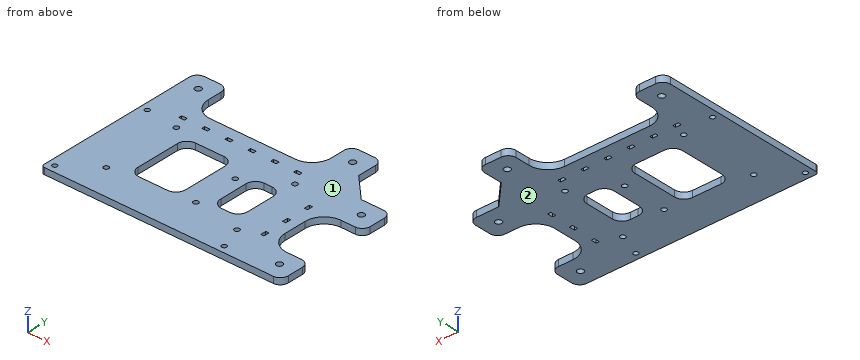
Autodesk Inventor part; units mm, degrees
ref_plane "YZ Plane" through (0, 0, 0) normal (1, 0, 0) x (0, 1, 0)
ref_plane "XZ Plane" through (0, 0, 0) normal (0, 1, 0) x (-1, 0, 0)
ref_plane "XY Plane" through (0, 0, 0) normal (0, 0, 1) x (1, 0, 0)
sketch "Szkic1" plane through (0, 0, 0) normal (0, 0, 1) x (1, 0, 0)
  line L0 (0, 53.1646) -> (0, 0)
  line L1 (0, 0) -> (98.9175, 0)
  line L2 (98.9175, 0) -> (98.9175, 1.2597)
  line L3 (98.9175, 1.2597) -> (101.455, 3.8466)
  line L4 (101.455, 3.8466) -> (101.455, 38.0126)
  line L5 (101.455, 38.0126) -> (98.9175, 40.5017)
  line L6 (98.9175, 40.5017) -> (98.9175, 50.7051)
  line L7 (98.9175, 50.7051) -> (96.4101, 53.1646)
  line L8 (96.4101, 53.1646) -> (0, 53.1646)
  circle A0 centre (96.3111, 2.4061) radius 1.6
  circle A1 centre (15.0311, 50.6661) radius 1.6
  circle A2 centre (89.9611, 50.6661) radius 1.6
  circle A3 centre (13.7611, 2.4061) radius 1.6
  circle A4 centre (65.8311, 35.4261) radius 1.6
  circle A5 centre (65.8311, 7.4861) radius 1.6
  line L9 (-10, 93.1646) -> (141.455, 93.1646)
  line L10 (141.455, 93.1646) -> (141.455, -17)
  line L11 (141.455, -17) -> (-10, -17)
  line L12 (-10, -17) -> (-10, 93.1646)
  line L13 (107.455, 93.1646) -> (107.455, 61.1646)
  line L14 (107.455, 61.1646) -> (141.455, 61.1646)
  point P0 (-10, 13.9306)
  point P1 (7.9866, -17)
  dimension "d0" = 101.455
  dimension "d1" = 53.1646
  dimension "d2" = 98.9175
  dimension "d3" = 15.0311
  dimension "d4" = 2.4986
  dimension "d5" = 3.2
  dimension "d6" = 2.4986
  dimension "d7" = 8.9564
  dimension "d8" = 3.2
  dimension "d9" = 3.2
  dimension "d10" = 17.7386
  dimension "d11" = 65.8311
  dimension "d12" = 13.7611
  dimension "d13" = 2.4061
  dimension "d14" = 7.486
  dimension "d15" = 65.8311
  dimension "d16" = 2.4061
  dimension "d17" = 5.144
  dimension "d18" = 3.2
  dimension "d19" = 3.2
  dimension "d20" = 3.2
  dimension "d21" = 98.9175
  dimension "d22" = 1.2597
  dimension "d23" = 10.2034
  dimension "d24" = 34.166
  dimension "d33" = 40
  dimension "d34" = 40
  dimension "d35" = 17
  dimension "d36" = 10
  dimension "d37" = 34
  dimension "d38" = 32
extrude "Wyciągnięcie proste1" add sketch "Szkic1" along normal blind 4 contours L8 L7 L6 L5 L4 L3 L2 L1 L0 | L9 L13 L14 L10 L11 L12
chamfer "Faza1" distance 15 angle 45 1 edges at (107.455, 61.1646, 2)
sketch "Szkic2" plane through (0, 0, 4) normal (0, 0, 1) x (1, 0, 0)
  circle A0 centre (65.8311, 7.4861) radius 1.6
  circle A1 centre (15.0311, 50.6661) radius 1.6
  circle A2 centre (89.9611, 50.6661) radius 1.6
  circle A3 centre (13.7611, 2.4061) radius 1.6
  circle A4 centre (65.8311, 35.4261) radius 1.6
  circle A5 centre (96.3111, 2.4061) radius 1.6
  line L0 (-10, 93.1646) -> (-10, -17)
  line L1 (-10, -17) -> (141.455, -17)
  line L2 (141.455, -17) -> (141.455, 61.1646)
  line L3 (141.455, 61.1646) -> (122.455, 61.1646)
  line L4 (107.455, 76.1646) -> (122.455, 61.1646)
  line L5 (107.455, 76.1646) -> (107.455, 93.1646)
  line L6 (107.455, 93.1646) -> (-10, 93.1646)
  line L7 (10, 93.1646) -> (10, 67.1646)
  line L8 (10, 67.1646) -> (87.455, 67.1646)
  line L9 (87.455, 67.1646) -> (87.455, 93.1646)
  line L10 (107.455, 93.1646) -> (-10, 93.1646)
  line L11 (141.455, -17) -> (141.455, 61.1646)
  line L12 (141.455, 41.1646) -> (115.455, 41.1646)
  line L13 (115.455, 41.1646) -> (115.455, 3)
  line L14 (115.455, 3) -> (141.455, 3)
  line L15 (10, 60.1646) -> (13.5, 60.1646)
  line L16 (13.5, 60.1646) -> (13.5, 58.1646)
  line L17 (13.5, 58.1646) -> (10, 58.1646)
  line L18 (10, 58.1646) -> (10, 60.1646)
  line L19 (28, 58.1646) -> (24.5, 58.1646)
  line L20 (28, 60.1646) -> (28, 58.1646)
  line L21 (24.5, 60.1646) -> (28, 60.1646)
  line L22 (24.5, 58.1646) -> (24.5, 60.1646)
  line L23 (42.5, 58.1646) -> (39, 58.1646)
  line L24 (42.5, 60.1646) -> (42.5, 58.1646)
  line L25 (39, 60.1646) -> (42.5, 60.1646)
  line L26 (39, 58.1646) -> (39, 60.1646)
  line L27 (57, 58.1646) -> (53.5, 58.1646)
  line L28 (57, 60.1646) -> (57, 58.1646)
  line L29 (53.5, 60.1646) -> (57, 60.1646)
  line L30 (53.5, 58.1646) -> (53.5, 60.1646)
  line L31 (71.5, 58.1646) -> (68, 58.1646)
  line L32 (71.5, 60.1646) -> (71.5, 58.1646)
  line L33 (68, 60.1646) -> (71.5, 60.1646)
  line L34 (68, 58.1646) -> (68, 60.1646)
  line L35 (86, 58.1646) -> (82.5, 58.1646)
  line L36 (86, 60.1646) -> (86, 58.1646)
  line L37 (82.5, 60.1646) -> (86, 60.1646)
  line L38 (82.5, 58.1646) -> (82.5, 60.1646)
  line L39 (109.455, 41.1646) -> (107.455, 41.1646)
  line L40 (107.455, 41.1646) -> (107.455, 37.6646)
  line L41 (107.455, 37.6646) -> (109.455, 37.6646)
  line L42 (109.455, 37.6646) -> (109.455, 41.1646)
  line L43 (107.455, 25.6646) -> (107.455, 22.1646)
  line L44 (107.455, 22.1646) -> (109.455, 22.1646)
  line L45 (109.455, 22.1646) -> (109.455, 25.6646)
  line L46 (109.455, 25.6646) -> (107.455, 25.6646)
  line L47 (107.455, 10.1646) -> (107.455, 6.6646)
  line L48 (107.455, 6.6646) -> (109.455, 6.6646)
  line L49 (109.455, 6.6646) -> (109.455, 10.1646)
  line L50 (109.455, 10.1646) -> (107.455, 10.1646)
  line L51 (54.7961, 6.5361) -> (24.7961, 6.5361)
  line L52 (24.7961, 6.5361) -> (24.7961, 46.5361)
  line L53 (24.7961, 46.5361) -> (54.7961, 46.5361)
  line L54 (54.7961, 46.5361) -> (54.7961, 6.5361)
  line L55 (89.5711, 11.5361) -> (72.5711, 11.5361)
  line L56 (72.5711, 11.5361) -> (72.5711, 41.5361)
  line L57 (72.5711, 41.5361) -> (89.5711, 41.5361)
  line L58 (89.5711, 41.5361) -> (89.5711, 11.5361)
  point P0 (0, 0)
  point P1 (131.455, -7)
  point P2 (131.455, 51.1646)
  point P3 (97.455, 83.1646)
  point P4 (0, 83.1646)
  dimension "d42" = 20
  dimension "d43" = 20
  dimension "d44" = 20
  dimension "d45" = 20
  dimension "d46" = 26
  dimension "d47" = 26
  dimension "d50" = 3.5
  dimension "d51" = 2
  dimension "d52" = 7
  dimension "d55" = 14.5
  dimension "d62" = 2
  dimension "d63" = 3.5
  dimension "d64" = 6
  dimension "d67" = 15.5
  dimension "d74" = 40
  dimension "d75" = 30
  dimension "d78" = 10
  dimension "d79" = 10
  dimension "d80" = 10
  dimension "d81" = 10
  dimension "d82" = 10
  dimension "d83" = 10
  dimension "d84" = 10
  dimension "d85" = 10
  dimension "d93" = 52.07
  dimension "d94" = 11.035
  dimension "d95" = 48.26
  dimension "d96" = 4.13
  dimension "d98" = 30
  dimension "d99" = 17
  dimension "d100" = 48.26
  dimension "d101" = 30.48
  dimension "d102" = 9.13
  dimension "d103" = 6.74
extrude "Wyciągnięcie proste3" cut sketch "Szkic2" against normal through all contours L6 L9 L8 L7 | L14 L13 L12 L2 | L15 L16 L17 L18 | L19 L22 L21 L20 | L23 L26 L25 L24 | L27 L30 L29 L28 | L31 L34 L33 L32 | L35 L38 L37 L36 | L42 L41 L40 L39 | L46 L45 L44 L43 | L50 L49 L48 L47 | L51 L52 L53 L54 | L55 L56 L57 L58
fillet "Zaokrąglenie1" radius 12 4 edges at (115.455, 41.1646, 2) (115.455, 3, 2) (87.455, 67.1646, 2) (10, 67.1646, 2)
fillet "Zaokrąglenie1" radius 5 8 edges at (10, 93.1646, 2) (-10, 93.1646, 2) (87.455, 93.1646, 2) (107.455, 93.1646, 2) (141.455, 61.1646, 2) (141.455, 41.1646, 2) (141.455, 3, 2) (141.455, -17, 2)
hole "Otwór1" at (131.455, -7, 4) at (131.455, 51.1646, 4) at (97.455, 83.1646, 4) at (0, 83.1646, 4) direction (0, 0, -1) diameter 4 end through all
fillet "Zaokrąglenie2" radius 6 8 edges at (24.7961, 6.5361, 2) (24.7961, 46.5361, 2) (54.7961, 46.5361, 2) (54.7961, 6.5361, 2) (89.5711, 11.5361, 2) (89.5711, 41.5361, 2) (72.5711, 41.5361, 2) (72.5711, 11.5361, 2)
fillet "Zaokrąglenie2" radius 2 1 edges at (-10, -17, 2)
sketch "Szkic4" plane through (0, 0, 4) normal (0, 0, 1) x (1, 0, 0)
  arc A0 (-10, -15) -> (-8, -17) centre (-8, -15) ccw
  line L0 (-8, -17) -> (136.455, -17)
  arc A1 (136.455, -17) -> (141.455, -12) centre (136.455, -12) ccw
  line L1 (141.455, -12) -> (141.455, -2)
  arc A2 (141.455, -2) -> (136.455, 3) centre (136.455, -2) ccw
  line L2 (136.455, 3) -> (127.455, 3)
  arc A3 (115.455, 15) -> (127.455, 3) centre (127.455, 15) ccw
  line L3 (115.455, 15) -> (115.455, 29.1646)
  arc A4 (127.455, 41.1646) -> (115.455, 29.1646) centre (127.455, 29.1646) ccw
  line L4 (127.455, 41.1646) -> (136.455, 41.1646)
  arc A5 (136.455, 41.1646) -> (141.455, 46.1646) centre (136.455, 46.1646) ccw
  line L5 (141.455, 46.1646) -> (141.455, 56.1646)
  arc A6 (141.455, 56.1646) -> (136.455, 61.1646) centre (136.455, 56.1646) ccw
  line L6 (136.455, 61.1646) -> (122.455, 61.1646)
  line L7 (107.455, 76.1646) -> (122.455, 61.1646)
  line L8 (107.455, 76.1646) -> (107.455, 88.1646)
  arc A7 (107.455, 88.1646) -> (102.455, 93.1646) centre (102.455, 88.1646) ccw
  line L9 (102.455, 93.1646) -> (92.455, 93.1646)
  arc A8 (92.455, 93.1646) -> (87.455, 88.1646) centre (92.455, 88.1646) ccw
  line L10 (87.455, 88.1646) -> (87.455, 79.1646)
  arc A9 (75.455, 67.1646) -> (87.455, 79.1646) centre (75.455, 79.1646) ccw
  line L11 (75.455, 67.1646) -> (22, 67.1646)
  arc A10 (10, 79.1646) -> (22, 67.1646) centre (22, 79.1646) ccw
  line L12 (10, 79.1646) -> (10, 88.1646)
  arc A11 (10, 88.1646) -> (5, 93.1646) centre (5, 88.1646) ccw
  line L13 (5, 93.1646) -> (-5, 93.1646)
  arc A12 (-5, 93.1646) -> (-10, 88.1646) centre (-5, 88.1646) ccw
  line L14 (-10, 88.1646) -> (-10, -15)
  circle A13 centre (97.455, 83.1646) radius 2
  circle A14 centre (131.455, -7) radius 2
  circle A15 centre (131.455, 51.1646) radius 2
  circle A16 centre (0, 83.1646) radius 2
  line L15 (89.5711, 35.5361) -> (89.5711, 17.5361)
  arc A17 (83.5711, 11.5361) -> (89.5711, 17.5361) centre (83.5711, 17.5361) ccw
  line L16 (83.5711, 11.5361) -> (78.5711, 11.5361)
  arc A18 (72.5711, 17.5361) -> (78.5711, 11.5361) centre (78.5711, 17.5361) ccw
  line L17 (72.5711, 17.5361) -> (72.5711, 35.5361)
  arc A19 (78.5711, 41.5361) -> (72.5711, 35.5361) centre (78.5711, 35.5361) ccw
  line L18 (78.5711, 41.5361) -> (83.5711, 41.5361)
  arc A20 (89.5711, 35.5361) -> (83.5711, 41.5361) centre (83.5711, 35.5361) ccw
  line L19 (107.455, 22.1646) -> (107.455, 25.6646)
  line L20 (107.455, 25.6646) -> (109.455, 25.6646)
  line L21 (109.455, 25.6646) -> (109.455, 22.1646)
  line L22 (109.455, 22.1646) -> (107.455, 22.1646)
  line L23 (82.5, 60.1646) -> (86, 60.1646)
  line L24 (86, 60.1646) -> (86, 58.1646)
  line L25 (86, 58.1646) -> (82.5, 58.1646)
  line L26 (82.5, 58.1646) -> (82.5, 60.1646)
  line L27 (53.5, 60.1646) -> (57, 60.1646)
  line L28 (57, 60.1646) -> (57, 58.1646)
  line L29 (57, 58.1646) -> (53.5, 58.1646)
  line L30 (53.5, 58.1646) -> (53.5, 60.1646)
  line L31 (24.5, 60.1646) -> (28, 60.1646)
  line L32 (28, 60.1646) -> (28, 58.1646)
  line L33 (28, 58.1646) -> (24.5, 58.1646)
  line L34 (24.5, 58.1646) -> (24.5, 60.1646)
  line L35 (10, 58.1646) -> (10, 60.1646)
  line L36 (10, 60.1646) -> (13.5, 60.1646)
  line L37 (13.5, 60.1646) -> (13.5, 58.1646)
  line L38 (13.5, 58.1646) -> (10, 58.1646)
  line L39 (39, 60.1646) -> (42.5, 60.1646)
  line L40 (42.5, 60.1646) -> (42.5, 58.1646)
  line L41 (42.5, 58.1646) -> (39, 58.1646)
  line L42 (39, 58.1646) -> (39, 60.1646)
  line L43 (68, 60.1646) -> (71.5, 60.1646)
  line L44 (71.5, 60.1646) -> (71.5, 58.1646)
  line L45 (71.5, 58.1646) -> (68, 58.1646)
  line L46 (68, 58.1646) -> (68, 60.1646)
  line L47 (107.455, 37.6646) -> (107.455, 41.1646)
  line L48 (107.455, 41.1646) -> (109.455, 41.1646)
  line L49 (109.455, 41.1646) -> (109.455, 37.6646)
  line L50 (109.455, 37.6646) -> (107.455, 37.6646)
  line L51 (107.455, 6.6646) -> (107.455, 10.1646)
  line L52 (107.455, 10.1646) -> (109.455, 10.1646)
  line L53 (109.455, 10.1646) -> (109.455, 6.6646)
  line L54 (109.455, 6.6646) -> (107.455, 6.6646)
  line L55 (54.7961, 40.5361) -> (54.7961, 12.5361)
  arc A21 (48.7961, 6.5361) -> (54.7961, 12.5361) centre (48.7961, 12.5361) ccw
  line L56 (48.7961, 6.5361) -> (30.7961, 6.5361)
  arc A22 (24.7961, 12.5361) -> (30.7961, 6.5361) centre (30.7961, 12.5361) ccw
  line L57 (24.7961, 12.5361) -> (24.7961, 40.5361)
  arc A23 (30.7961, 46.5361) -> (24.7961, 40.5361) centre (30.7961, 40.5361) ccw
  line L58 (30.7961, 46.5361) -> (48.7961, 46.5361)
  arc A24 (54.7961, 40.5361) -> (48.7961, 46.5361) centre (48.7961, 40.5361) ccw
  circle A25 centre (65.8311, 7.4861) radius 1.6
  circle A26 centre (15.0311, 50.6661) radius 1.6
  circle A27 centre (89.9611, 50.6661) radius 1.6
  circle A28 centre (13.7611, 2.4061) radius 1.6
  circle A29 centre (65.8311, 35.4261) radius 1.6
  circle A30 centre (96.3111, 2.4061) radius 1.6
  point P0 (0, 0)
  point P1 (-5.5, 53.1646)
  point P2 (-5.5, -12.5)
  point P3 (101.455, -12.5)
  dimension "d105" = 40
  dimension "d106" = 40
  dimension "d107" = 4.5
  dimension "d108" = 4.5
  dimension "d109" = 4.5
  dimension "d110" = 4.5
hole "Otwór2" at (-5.5, 53.1646, 4) at (-5.5, -12.5, 4) at (101.455, -12.5, 4) direction (0, 0, -1) diameter 3 end through all
equation "\"d47\" = d46"
equation "\"d94\" = -0.5 * d75 + 0.5 * d93"
equation "\"d96\" = -0.5 * d74 + 0.5 * d95"
equation "\"d102\" = -0.5 * d98 + 0.5 * d100"
equation "\"d103\" = -0.5 * d99 + 0.5 * d101"
properties part number "3DP_PLA_Controller_Case_Bottom"
Geometry check sheet. Reference: the model listing, model coordinates, mm. Face numbers are marked on the shaded views. Give positions to 0.01 mm unless a question says otherwise; leave off trailing zeros. Write each loop counter-clockwise with the first axis right and the second up, starting at its lowest first coordinate (ties: lowest second). Pieces come first, ordered by that corner, then holes. Notation, with made-up numbers: M -23,39.25 L -14,39.25 A17 ccw -14,65.25 Z; hole C 81.25,24.25 d5. An arc over 180 degrees is marked long. One line per question, with ' | ' between items.
1. Cross-section at B-B (x = 113.5). Enter the section's corners in (y, z), plus the area to 3 significant figures.
Ans:
outline: M -17,0 L 70.12,0 L 70.12,4 L -17,4 Z | area: 348 mm2
2. Scan lines: line 1 along X through (y, z) = (83, 0.55) (3 decimals); line 2 along X through (y, z) = (24, 2.7) (3 decimals); line 3 along X through (y, z) = (28.5, 2.2) (3 decimals). Record each from-to range of solid material in increasing order. Write a range as from..to.
Ans:
line 1: -10..-1.993, 1.993..10, 87.455..95.462, 99.448..107.455 | line 2: -10..24.796, 54.796..72.571, 89.571..107.455, 109.455..115.455 | line 3: -10..24.796, 54.796..72.571, 89.571..115.455
3. Mould release check, pull along Z, two halves, no side actions. Record for the marked faces 1 and 2: released by +Z, released by -Z, zero draft, split by the parting line, or undercut.
Ans:
face 1: released by +Z | face 2: released by -Z
4. Cross-section at A-A (x = 0). Enter the section's corners in (y, z), plus the area to 3 significant figures.
Ans:
outline: M -17,0 L 81.16,0 L 81.16,4 L -17,4 Z; M 85.16,0 L 93.16,0 L 93.16,4 L 85.16,4 Z | area: 425 mm2
5. Gauge pin test, flat ends, axial feed: pin 1 (2 mm diameter, centred on y = 59, z = 2.5, fed in from +X); pin 2 (4 mm diameter, centred on x = 101.455, y = -12.5, fed in from -Z); pin 3 (1.8 mm diameter, centred on x = 25.5, z = 2.5, fed in from +Y); pin 4 (1 mm diameter, centred on x = 85, z = 2, fed in from +Y). Record the tip position at first contact, or that the pin passes through.
Ans:
pin 1: x = 141.11 | pin 2: z = 0 | pin 3: y = 67.16 | pin 4: y = 72.6
6. Cross-section at C-C (z = 2.25). Count the separate pieces of the cut face and the enclosed holes in it, plus the area to 3 significant figures.
Ans:
separate pieces: 1 | enclosed holes: 24 | area: 11,000 mm2
